The model under review builds one solid part; all positions refer to its coordinate system, in mm. Round coordinates to 2 decimals unless told otherwise and drop trailing zeros. Loops run counter-clockwise (first coordinate to the right, second up) from the corner with the lowest first, then second, coordinate; pieces in that order, holes last. Notation, with made-up numbers: (32.5, 18) -> (64.5, 18) arc R22 cw to (64.5, 37) -> close; hole circle Ø7 at (-21, -7). An arc over 180 degrees is marked (long way). Return JSON: item names as keys, results as strings. Group by question number.
```python
from build123d import *

# Parameters (mm, degrees)
SKETCH1_W               = 200
SKETCH1_H               = 50.7
SKETCH1_W_2             = 240.661854396
SKETCH1_H_2             = 47.7
BOSS_EXTRUDE1_DEPTH     = 3.3
SKETCH2_R               = 1.5
CUT_EXTRUDE1_DEPTH      = 453.205952877
CUT_EXTRUDE2_DEPTH      = 455.953272433
CUT_EXTRUDE2_DEPTH_BACK = 455.953272433
SKETCH3_W               = 24.5
SKETCH3_H               = 54
SKETCH4_W               = 26.984189883
SKETCH4_H               = 54
CUT_EXTRUDE3_DEPTH      = 10
SKETCH6_W               = 56.727923661
SKETCH6_H               = 30
CUT_EXTRUDE4_DEPTH      = 10
SKETCH7_W               = 20
SKETCH7_H               = 3.3
BOSS_EXTRUDE2_DEPTH     = 3.3


with BuildPart() as part:
    # Sketch1 → Boss-Extrude1 (new body)
    with BuildSketch(Plane.XY):
        Polygon((25.5, 1), (25.5, -13), (25.5, -225), (25.5, -265), (65.632913627, -265), (123.748117859, -265), (323.748117859, -265), (323.748117859, 30), (83.086263463, 30), (25.5, 30), align=None)
        with Locations((223.748117859, -290.35)):
            Rectangle(SKETCH1_W, SKETCH1_H)
        with Locations((203.417190661, 53.85)):
            Rectangle(SKETCH1_W_2, SKETCH1_H_2)
    extrude(amount=BOSS_EXTRUDE1_DEPTH)

    # Sketch2 → Cut-Extrude1 (cut, through all)
    with BuildSketch(Plane(origin=(0, 0, 0), x_dir=(-1, 0, 0), z_dir=(0, 0, -1))):
        with Locations((-150.216261358, 72.7)):
            Circle(SKETCH2_R)
        with Locations((-124.61492379, 72.7)):
            Circle(SKETCH2_R)
        with Locations((-205.394208158, -310.7)):
            Circle(SKETCH2_R)
        with Locations((-185.309760184, -310.7)):
            Circle(SKETCH2_R)
    extrude(amount=-CUT_EXTRUDE1_DEPTH, mode=Mode.SUBTRACT)

    # Sketch3 → Cut-Extrude2 (cut, two sides: drawn at the far end of the back side and taken through both)
    with BuildSketch(Plane(origin=(119.391473557, 0, 256.035841294), x_dir=(0.9063077870366519, 0, -0.42261826174069517), z_dir=(0.42261826174069517, 0, 0.9063077870366519)).offset(-CUT_EXTRUDE2_DEPTH_BACK)):
        with Locations((281.209458836, -119)):
            Rectangle(SKETCH3_W, SKETCH3_H)
    extrude(amount=CUT_EXTRUDE2_DEPTH + CUT_EXTRUDE2_DEPTH_BACK, mode=Mode.SUBTRACT)

    # Sketch4 → Cut-Extrude3 (cut)
    with BuildSketch(Plane(origin=(0, 0, 0), x_dir=(-1, 0, 0), z_dir=(0, 0, -1))):
        with Locations((-310.256022917, -119)):
            Rectangle(SKETCH4_W, SKETCH4_H)
    extrude(amount=-CUT_EXTRUDE3_DEPTH, mode=Mode.SUBTRACT)

    # Sketch6 → Cut-Extrude4 (cut)
    with BuildSketch(Plane.XY.offset(3.3)):
        with Locations((53.863961831, 15)):
            Rectangle(SKETCH6_W, SKETCH6_H)
    extrude(amount=-CUT_EXTRUDE4_DEPTH, mode=Mode.SUBTRACT)

    # Sketch7 → Boss-Extrude2 (add)
    with BuildSketch(Plane(origin=(0, 0, 0), x_dir=(-1, 0, 0), z_dir=(0, 0, -1))):
        with Locations((-193.748117858, -317.35)):
            Rectangle(SKETCH7_W, SKETCH7_H)
        with Locations((-153.748117858, -317.35)):
            Rectangle(SKETCH7_W, SKETCH7_H)
        with Locations((-113.748117859, 79.35)):
            Rectangle(SKETCH7_W, SKETCH7_H)
        with Locations((-153.748117859, 79.35)):
            Rectangle(SKETCH7_W, SKETCH7_H)
        with Locations((-233.748117858, -317.35)):
            Rectangle(SKETCH7_W, SKETCH7_H)
        with Locations((-193.748117859, 79.35)):
            Rectangle(SKETCH7_W, SKETCH7_H)
        with Locations((-273.748117858, -317.35)):
            Rectangle(SKETCH7_W, SKETCH7_H)
        with Locations((-233.748117859, 79.35)):
            Rectangle(SKETCH7_W, SKETCH7_H)
        with Locations((-313.748117858, -317.35)):
            Rectangle(SKETCH7_W, SKETCH7_H)
        with Locations((-273.748117859, 79.35)):
            Rectangle(SKETCH7_W, SKETCH7_H)
        with Locations((-313.748117859, 79.35)):
            Rectangle(SKETCH7_W, SKETCH7_H)
    extrude(amount=-BOSS_EXTRUDE2_DEPTH)


solid = part.part
```
1. We need section A-A, the plane z = 0.95. Give the number of separate pieces and of enclosed holes in the cut face, then the cut area to 3 significant figures.
2. We need section B-B, the plane x = 66.5. Write out the cut boundary in (y, z), then the cut area to 4 significant figures.
3. Wall thickness on line 1 (X direction, y = -310.7, z = 1.4); line 2 (X direction, y = 72.7, z = 0.85); line 3 (Y direction, x = 173.5, z = 1.3): over which ranges is each line inside the solid? List them lowest first.
4. For P1, Ø1.6, axis at y = 80, z = 1, coming from the -X side; P2, Ø0.9, axis at x = 82.5, z = 2, coming from the +Y side; P3, Ø1.6, axis at x = 173.5, z = 1.5, coming from the -Y side, all flat-tipped, find the tip position at first contact; note any pin that passes through.
Check sheet entries:
{
 "1": {"separate pieces": "1", "enclosed holes": "4", "area": "107,000 mm²"},
 "2": {"outline": "(-265, 0) -> (0, 0) -> (0, 3.3) -> (-265, 3.3) -> close", "area": "874.5 mm²"},
 "3": {"line 1": "x = 123.75 to 183.81, 186.81 to 203.89, 206.89 to 323.75", "line 2": "x = 83.09 to 123.11, 126.11 to 148.72, 151.72 to 323.75", "line 3": "y = -315.7 to 77.7"},
 "4": {"P1": "stops at x = 103.75", "P2": "stops at y = 30", "P3": "stops at y = -315.7"}
}
